The listing builds one solid part. Answer for the finished solid, in the listing's coordinates (mm). A direction names the side the tool comes from. Give positions to 0.01 mm unless a question says otherwise; leave off trailing zeros. Order: outer loops, then holes, each group sorted by start corner. A loop starts at its lowest first (then second) coordinate and runs counter-clockwise, first axis right, second up. Notation, with made-up numbers: (78, 59) -> (100, 59) arc R20 cw to (100, 79) -> close; hole circle Ø2 at (24.25, -21.75). An arc over 180 degrees is marked (long way). One line per question, with ' | ' between items. Start each with the question number.
```python
from build123d import *

# Parameters (mm, degrees)
BOSS_EXTRUDE1_DEPTH                                = 9.525
FILLET1_R                                          = 1.5875
CSK_FOR_10_FLAT_HEAD_MACHINE_SCREW_100_D           = 5.1054
CSK_FOR_10_FLAT_HEAD_MACHINE_SCREW_100_CSINK_D     = 9.779
CSK_FOR_10_FLAT_HEAD_MACHINE_SCREW_100_CSINK_ANGLE = 100


with BuildPart() as part:
    # Sketch1 → Boss-Extrude1 (new body, symmetric)
    with BuildSketch(Plane(origin=(0, 0, 0), x_dir=(0, 0, -1), z_dir=(1, 0, 0))):
        with BuildLine():
            Line((-13.6525, -2.54), (8.5725, -2.54))
            Line((8.5725, -2.54), (8.5725, -78.74))
            ThreePointArc((8.5725, -78.74), (28.76659153, -92.233260572), (33.504794539, -68.412705461))
            Line((33.504794539, -68.412705461), (29.912692091, -72.004807909))
            ThreePointArc((29.912692091, -72.004807909), (26.822559693, -87.539952547), (13.6525, -78.74))
            Line((13.6525, -78.74), (13.6525, 2.54))
            Line((13.6525, 2.54), (-13.6525, 2.54))
            Line((-13.6525, 2.54), (-13.6525, -2.54))
        make_face()
    extrude(amount=BOSS_EXTRUDE1_DEPTH, both=True)

    # Fillet1
    fillet1_edges = [part.edges().sort_by_distance(p)[0] for p in [
        (0, -72.004807909, -29.912692091),
        (0, -68.412705461, -33.504794539),
        (0, -2.54, -8.5725),
        (0, -2.54, 13.6525),
        (0, 2.54, 13.6525),
        (0, 2.54, -13.6525),
    ]]
    fillet(fillet1_edges, radius=FILLET1_R)

    # CSK for #10 Flat Head Machine Screw (100)1 (through all)
    with Locations(Plane(origin=(0, 2.54, 2.54), x_dir=(0, 0, 1), z_dir=(0, 1, 0))):
        with Locations((0, 0)):
            CounterSinkHole(CSK_FOR_10_FLAT_HEAD_MACHINE_SCREW_100_D / 2, CSK_FOR_10_FLAT_HEAD_MACHINE_SCREW_100_CSINK_D / 2, counter_sink_angle=CSK_FOR_10_FLAT_HEAD_MACHINE_SCREW_100_CSINK_ANGLE)


solid = part.part
```
(1) Consider line 1 (Z direction, x = 4, y = -78.74); line 2 (X direction, y = -0.7, z = 2.54) (3 decimals); line 3 (Z direction, x = 6, y = -33). Determine where each line is inside the solid, lowest interval first.
(2) The part is cut by section A-A on z = 2.54. Determine the outline of the cut face in (x, y) (1 decimal), plus the area to 3 significant figures.
(3) Determine the mould class of faces 3 (the face through (0.133, -87.696, -26.421)), 4 (the face through (0.13, -69.14, -33.51)), 5 (the face through (0.133, -71.988, -30.493)), 6 (the face through (9.525, -49, -12)) for opening direction Y: pulls with the +Y half, pulls with the -Y half, needs draft (parallel to the pull), parting line crosses it, or undercut.
(4) The part is cut by section D-D on z = -27. Determine the outline of the cut face in (x, y) (3 decimals), plus the area to 3 significant figures.
(5) For faces 1 (the face through (0.13, -92.67, -27.56)), 2 (the face through (0, -41, -8.572)), determine the directions among +Z, -Z, +X, -X, +Y, -Y from which every point of the face is accessible in a straight line to the end or side of a thin tool.
(6) Given P1, Ø5, axis at x = -1, z = -15.5, coming from the -Y side; P2, Ø1.5, axis at x = -4.5, y = -35.5, coming from the -Z side; P3, Ø9.5, axis at x = 0, y = -42, coming from the +Z side, each flat-ended and moving along its own axis, determine where each tip first touches the part or whether it passes through.
(7) The part is cut by section C-C on y = -9. Determine the outline of the cut face in (x, z) (1 decimal), plus the area to 3 significant figures.
Result sheet:
1) line 1: z = -37.78 to -32.7, -13.65 to -8.57 | line 2: x = -9.525 to -2.553, 2.553 to 9.525 | line 3: z = -13.65 to -8.57
2) outline: (-9.5, -2.5) -> (-2.6, -2.5) -> (-2.6, 0.6) -> (-4.9, 2.5) -> (-9.5, 2.5) -> close; (2.6, -2.5) -> (9.5, -2.5) -> (9.5, 2.5) -> (4.9, 2.5) -> (2.6, 0.6) -> close | area: 66.3 mm^2
3) face 3: undercut | face 4: pulls with the +Y half | face 5: undercut | face 6: needs draft
4) outline: (-9.525, -92.836) -> (9.525, -92.836) -> (9.525, -87.464) -> (-9.525, -87.464) -> close | area: 102 mm^2
5) face 1: +X, -X | face 2: +Z, +X, -X, -Y
6) P1: stops at y = -92.4 | P2: stops at z = -13.65 | P3: stops at z = -8.57
7) outline: (-9.5, -13.7) -> (9.5, -13.7) -> (9.5, -8.6) -> (-9.5, -8.6) -> close | area: 96.8 mm^2
